```python
from build123d import *

# Parameters (mm, degrees)
F0_W     = 38.1
F0_H     = 25.4
F1_DEPTH = 3.175
F3_DEPTH = 6.35
F4_R     = 1.5875
F5_DEPTH = 3.175
F6_SIZE  = 1


with BuildPart() as f1:
    # F0 (on Right) → F1 (new body)
    with BuildSketch(Plane.YZ):
        Rectangle(F0_W, F0_H)
    extrude(amount=F1_DEPTH)

    # F2 (on face) → F3 (join)
    with BuildSketch(Plane.YZ.offset(3.175)):
        with BuildLine():
            ThreePointArc((4.064, 0), (0, -4.064), (-4.064, 0))
            Line((-4.064, 0), (-4.064, 3.175))
            Line((-4.064, 3.175), (-7.239, 3.175))
            Line((-7.239, 3.175), (-7.239, 0))
            ThreePointArc((-7.239, 0), (0, -7.239), (7.239, 0))
            Line((7.239, 0), (7.239, 3.175))
            Line((7.239, 3.175), (4.064, 3.175))
            Line((4.064, 3.175), (4.064, 0))
        make_face()
    extrude(amount=F3_DEPTH)

    # F4 (on face) → F5 (cut, through all)
    with BuildSketch(Plane.YZ.offset(3.175)):
        with Locations((-14.986, 0)):
            Circle(F4_R)
        with Locations((14.986, 0)):
            Circle(F4_R)
        Circle(F4_R)
    extrude(amount=-F5_DEPTH, mode=Mode.SUBTRACT)

    # F6
    f6_edges = [f1.edges().sort_by_distance(p)[0] for p in [
        (6.35, -4.064, 3.175),
        (6.35, 4.064, 3.175),
        (3.175, -19.05, 0),
        (3.175, 0, 12.7),
        (3.175, 19.05, 0),
        (3.175, 0, -12.7),
        (3.175, 0, -7.239),
        (3.175, -7.239, 1.5875),
        (3.175, 7.239, 1.5875),
    ]]
    chamfer(f6_edges, length=F6_SIZE)


solid = f1.part
```
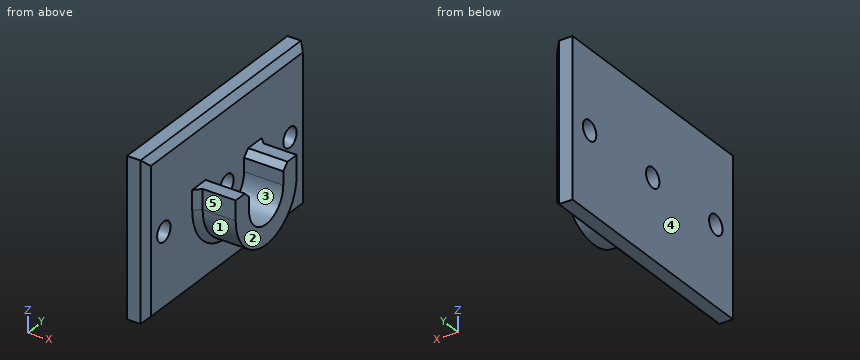
Could you check a few things on this model? Use its own coordinates, in mm. Face numbers are marked on the shaded views. A direction names the side the tool comes from. Round coordinates to 2 decimals unless told otherwise and drop trailing zeros. Write each loop counter-clockwise with the first axis right and the second up, starting at its lowest first coordinate (ties: lowest second). Pieces come first, ordered by that corner, then holes. Notation, with made-up numbers: M 1.25,-34 L 33.25,-34 A18 cw 33.25,-27 Z; hole C -31.5,79 d7. An arc over 180 degrees is marked long. Write each question's results on one line, items separated by ' | '. Start each with the question number.
1. Imagine slicing it at C-C on x = 1.25. Count the separate pieces of the cut face and the enclosed holes in it, and give its area (3 significant figures).
2. Imagine slicing it at D-D on y = 9. List the corners of the cut face in (x, z) for me (3 decimals).
3. I'm going to push flat-ended pins straight in: pin 1 Ø1.6 at (x, z) = (5.5, 2) entering from -Y; pin 2 Ø1.6 at (x, y) = (6, -7.5) entering from +Z (3 decimals); pin 3 Ø3 at (y, z) = (14.986, 0) entering from -X; pin 4 Ø1.6 at (x, z) = (7.5, 1) entering from +Y. Where does each tip first touch, or does it pass through?
4. I need wall thicknesses on L1, parallel to Y at x = 2.75, z = -0.25 (3 decimals); L2, parallel to X at y = -15.5, z = 8 (3 decimals); L3, parallel to Y at x = 8.75, z = 2. Which ranges of each line are inside material? Lowest first, please. Write a range as from..to.
5. Imagine slicing it at A-A on y = 0. List the corners of the cut face in (x, z) for me (1 decimal).
6. Imagine slicing it at B-B on x = 4.75. List the corners of the cut face in (y, z) for me (3 decimals).
7. Thinking about a two-plate mould opening in Y: for the marked faces 1, 2 and 3, which applies, +Y half, -Y half, draft (parallel to the pull), parting line (faces both ways), or undercut?
8. On a 3-axis mill with a long thin cutter (end or side, diameter ignored), from which of +Z, -Z, +X, -X, +Y, -Y can I reach the whole of each face in a straight line? I mean the marked faces 4 and 5. Say none if no direction works.
Result sheet:
1) separate pieces: 1 | enclosed holes: 3 | area: 944 mm^2
2) outline: M 0,-12.7 L 2.175,-12.7 L 3.175,-11.7 L 3.175,11.7 L 2.175,12.7 L 0,12.7 Z
3) pin 1: stops at y = -7.24 | pin 2: stops at z = 3.175 | pin 3: passes through | pin 4: stops at y = 7.24
4) L1: y = -18.475..-16.554, -13.418..-1.568, 1.568..13.418, 16.554..18.475 | L2: x = 0..3.175 | L3: y = -7.24..-4.06, 4.06..7.24
5) outline: M 0,-12.7 L 2.2,-12.7 L 3.2,-11.7 L 3.2,-8.2 L 4.2,-7.2 L 9.5,-7.2 L 9.5,-4.1 L 3.2,-4.1 L 3.2,-1.6 L 0,-1.6 Z; M 0,1.6 L 3.2,1.6 L 3.2,11.7 L 2.2,12.7 L 0,12.7 Z
6) outline: M -7.239,0 A7.239 ccw 7.239,0 L 7.239,3.175 L 5.064,3.175 L 4.064,2.175 L 4.064,0 A4.064 cw -4.064,0 L -4.064,2.175 L -5.064,3.175 L -7.239,3.175 Z
7) face 1: parting line | face 2: draft | face 3: undercut
8) face 4: +Z, -Z, -X, +Y, -Y | face 5: +Z, -Z, +X, -Y
